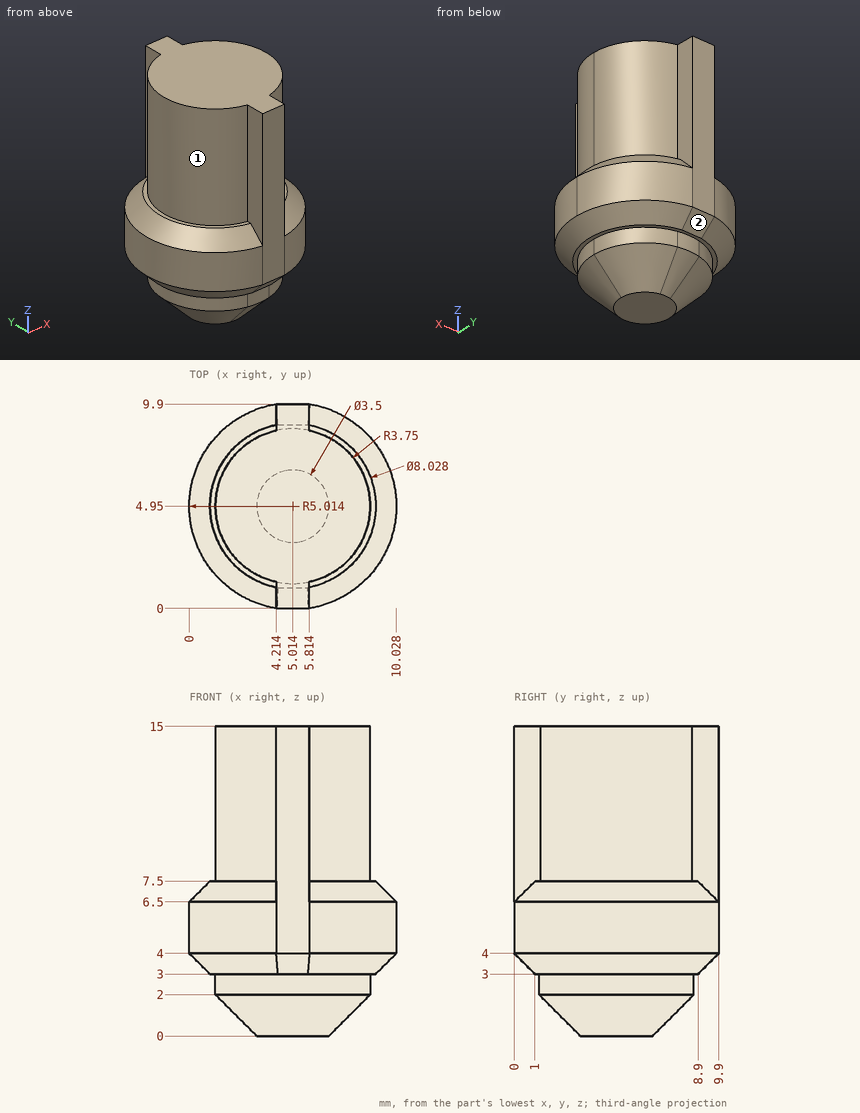
Can you work these out from the drawing? Everything is in mm from the part's minimum corner. A direction names the side the tool comes from. Coordinates: 2 decimals unless noted, no trailing zeros.
1) Which directions (+Z, -Z, +X, -X, +Y, -Y) give clear straight access to the entire face, cutting with the end or side of a thin tool? Please do the marked faces 1 and 2.
2) For pin 1 (1.4 mm diameter, centred on y = 9.5, z = 11.5, fed in from -X); pin 2 (1.5 mm diameter, centred on x = 1, y = 4, fed in from -Z) (1 decimal); pin 3 (4 mm diameter, centred on y = 3.5, z = 12, fed in from +X), each with a flat end and sliding along its axis, tell me the tip position at first contact or that it passes through.
3) I need wall thicknesses on probe 1 along Z at (x, y) = (6.75, 1.5); probe 2 along X at (y, z) = (8, 4.5) (1 decimal); probe 3 along Z at (x, y) = (9.75, 5.75). Which ranges of each line are inside material? Lowest first, please.
Completed:
1. face 1: +Z, -X
1. face 2: -Z, +X, -X, +Y
2. pin 1: stops at x = 4.21
2. pin 2: stops at z = 1.6
2. pin 3: stops at x = 8.76
3. probe 1: z = 3 to 7.5
3. probe 2: x = 1 to 9
3. probe 3: z = 3.79 to 6.71
